Here's how the part is built. I have some questions about the finished solid (model axes, mm). Face numbers are marked on the shaded views. A direction names the side the tool comes from. Coordinates: 2 decimals unless noted, no trailing zeros. Order: outer loops, then holes, each group sorted by start corner. A loop starts at its lowest first (then second) coordinate and runs counter-clockwise, first axis right, second up. Notation, with made-up numbers: (87, -29) - (111, -29) arc R24 cw to (111, -10) - close; hole circle Ø7 at (21, -6). An arc over 180 degrees is marked (long way). Answer in a Markdown table with one row per item. Add a question column.
Item 1: I want a section at C-C (z = -1). Please give me the cut outline in (x, y) (3 decimals), plus the area to 3 significant figures.
Item 2: Will these pins go through, and if not, where does the flat tip stop? pin 1 Ø3 at (y, z) = (28.5, -2.5) entering from +X; pin 2 Ø4.5 at (x, z) = (69, -3.5) entering from +Y; pin 3 Ø4.5 at (x, z) = (69, -3.5) entering from -Y.
Item 3: If I drill on line 1 along X through (y, z) = (33, -6.75); line 2 along Y through (x, z) = (66.75, -7); line 3 along Y through (x, z) = (68, -6.5), over which ranges is the centre line in solid material (lowest first)? Write a range as from..to.
Item 4: Thinking about a two-plate mould opening in X: for the marked faces 3, 4 and 5, which applies, +X half, -X half, draft (parallel to the pull), parting line (faces both ways), or undercut?
Item 5: I want a section at D-D (y = 28.75). Please give me the cut outline in (x, z), plus the area to 3 significant figures.
Item 6: On a 3-axis mill with a long thin cutter (end or side, diameter ignored), from which of +Z, -Z, +X, -X, +Y, -Y can I reach the whole of each face in a straight line? I mean the marked faces 1 and 2. Say none if no direction works.
Item 7: I want a section at B-B (y = 31.75). Please give me the cut outline in (x, z).
Item 8: I want a section at A-A (x = 69.5). Please give me the cut outline in (y, z), plus the area to 3 significant figures.
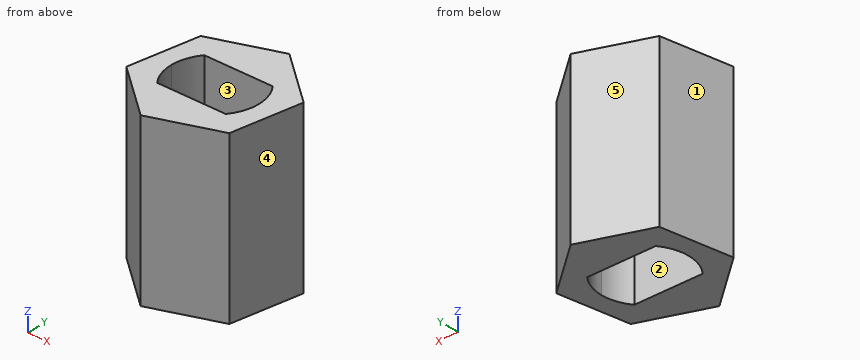
Autodesk Inventor part; units mm, degrees
ref_plane "YZ Plane" through (0, 0, 0) normal (1, 0, 0) x (0, 1, 0)
ref_plane "XZ Plane" through (0, 0, 0) normal (0, 1, 0) x (-1, 0, 0)
ref_plane "XY Plane" through (0, 0, 0) normal (0, 0, 1) x (1, 0, 0)
ref_plane "Arbeitsebene1" through (0, 0, 0) normal (0, 0, 1) x (1, 0, 0)
sketch "Skizze1" plane through (0, 0, 0) normal (0, 0, 1) x (1, 0, 0)
  line L0 (66.6303, 35.3317) -> (67.8519, 35.7763)
  circle A0 centre (68.575, 31.8892) radius 5.5
  line L1 (65.3022, 34.6354) -> (69.3169, 36.0967)
  line L2 (69.3169, 36.0967) -> (72.5897, 33.3504)
  line L3 (72.5897, 33.3504) -> (71.8478, 29.143)
  line L4 (71.8478, 29.143) -> (67.8331, 27.6817)
  line L5 (67.8331, 27.6817) -> (64.5603, 30.428)
  line L6 (64.5603, 30.428) -> (65.3022, 34.6354)
  arc A1 (66.575, 33.3892) -> (66.075, 31.8892) centre (68.575, 31.8892) ccw
  line L7 (70.575, 33.3892) -> (66.575, 33.3892)
  arc A2 (71.075, 31.8892) -> (70.575, 33.3892) centre (68.575, 31.8892) ccw
  arc A3 (70.575, 30.3892) -> (71.075, 31.8892) centre (68.575, 31.8892) ccw
  line L8 (66.575, 30.3892) -> (70.575, 30.3892)
  arc A4 (66.075, 31.8892) -> (66.575, 30.3892) centre (68.575, 31.8892) ccw
  arc A5 (66.5256, 33.4892) -> (65.975, 31.8892) centre (68.575, 31.8892) ccw
  arc A6 (65.975, 31.8892) -> (66.5256, 30.2892) centre (68.575, 31.8892) ccw
  line L9 (66.5256, 30.2892) -> (70.6244, 30.2892)
  arc A7 (70.6244, 30.2892) -> (71.175, 31.8892) centre (68.575, 31.8892) ccw
  arc A8 (71.175, 31.8892) -> (70.6244, 33.4892) centre (68.575, 31.8892) ccw
  line L10 (70.6244, 33.4892) -> (66.5256, 33.4892)
  point P0 (0, 0)
  dimension "d0" = 0.2
  dimension "d3" = 0.1
extrude "Extrusion1" add sketch "Skizze1" against normal blind 10 contours L1 L2 L3 L4 L5 L6
properties part number "11_Motor_to_Cassette_Clutch"
Values follow:
| question | item | result |
|---|---|---|
| 1 | outline | (64.56, 30.428) - (67.833, 27.682) - (71.848, 29.143) - (72.59, 33.35) - (69.317, 36.097) - (65.302, 34.635) - close; hole (65.975, 31.889) arc R2.6 ccw to (66.526, 30.289) - (70.624, 30.289) arc R2.6 ccw to (71.175, 31.889) arc R2.6 ccw to (70.624, 33.489) - (66.526, 33.489) arc R2.6 ccw to start |
| 1 | area | 31.9 mm^2 |
| 2 | pin 1 | stops at x = 72 |
| 2 | pin 2 | stops at y = 36.1 |
| 2 | pin 3 | stops at y = 27.68 |
| 3 | line 1 | x = 65.01..66.22, 70.93..72.53 |
| 3 | line 2 | y = 28.59..30.29, 33.49..35.16 |
| 3 | line 3 | y = 27.74..30.29, 33.49..35.62 |
| 4 | face 3 | undercut |
| 4 | face 4 | +X half |
| 4 | face 5 | -X half |
| 5 | outline | (66.56, -10) - (70.77, -10) - (70.77, 0) - (66.56, 0) - close |
| 5 | area | 42.1 mm^2 |
| 6 | face 1 | +Z, -Z, -X, +Y |
| 6 | face 2 | +Z, -Z |
| 7 | outline | (64.79, -10) - (65.98, -10) - (65.98, 0) - (64.79, 0) - close; (71.17, -10) - (72.31, -10) - (72.31, 0) - (71.17, 0) - close |
| 8 | outline | (28.29, -10) - (30.29, -10) - (30.29, 0) - (28.29, 0) - close; (33.49, -10) - (35.94, -10) - (35.94, 0) - (33.49, 0) - close |
| 8 | area | 44.5 mm^2 |
